Geometry check sheet. Reference: drawing and pictorial views, mm from the part's lowest x, y, z. A direction names the side the tool comes from. Coordinates: 2 decimals unless noted, no trailing zeros. Loops run counter-clockwise (first coordinate to the right, second up) from the corner with the lowest first, then second, coordinate; pieces in that order, holes last.
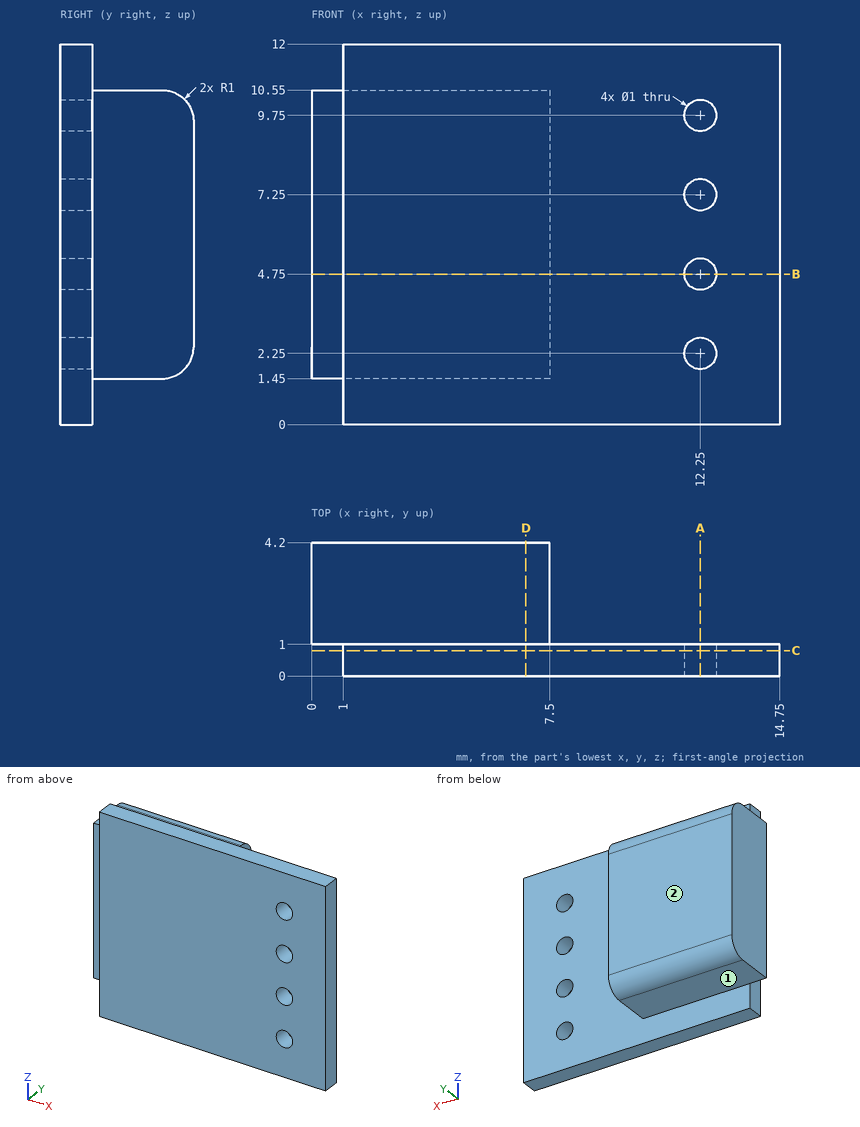
1) Access from +Z, -Z, +X, -X, +Y, -Y to the whole of each face (thin tool, end or side, straight path). Record for the marked faces 1 and 2.
Data:
face 1: -Z, +X, -X, +Y
face 2: +Z, -Z, +X, -X, +Y
2) Depth check by flat-ended pin: pin 1 (0.5 mm diameter, centred on x = 0.5, z = 6.5, fed in from -Y); pin 2 (2.5 mm diameter, centred on x = 4, y = 2.5, fed in from -Z); pin 3 (1 mm diameter, centred on x = 6.5, y = 4, fed in from -Z); pin 4 (1.1 mm diameter, centred on x = 4.5, y = 1.5, fed in from +Z). Enter the tip coordinate at first touch or a pass-through.
Data:
pin 1: stops at y = 1
pin 2: stops at z = 1.45
pin 3: stops at z = 1.5
pin 4: stops at z = 12
3) Material ranges on probe 1 along X at (y, z) = (0.5, 4.75); probe 2 along Z at (x, y) = (0.5, 1.15); probe 3 along Y at (x, z) = (13.5, 10.75), recorded low to high.
Data:
probe 1: x = 1 to 11.75, 12.75 to 14.75
probe 2: z = 1.45 to 10.55
probe 3: y = 0 to 1
4) Section check A-A on x = 12.25. Record the cut outline in (y, z).
Data:
outline: (0, 0) - (1, 0) - (1, 1.75) - (0, 1.75) - close; (0, 2.75) - (1, 2.75) - (1, 4.25) - (0, 4.25) - close; (0, 5.25) - (1, 5.25) - (1, 6.75) - (0, 6.75) - close; (0, 7.75) - (1, 7.75) - (1, 9.25) - (0, 9.25) - close; (0, 10.25) - (1, 10.25) - (1, 12) - (0, 12) - close
5) Section check C-C on y = 0.8. Record the cut outline in (x, z).
Data:
outline: (1, 0) - (14.75, 0) - (14.75, 12) - (1, 12) - close; hole circle Ø1 at (12.25, 2.25); hole circle Ø1 at (12.25, 4.75); hole circle Ø1 at (12.25, 7.25); hole circle Ø1 at (12.25, 9.75)
6) Section check D-D on x = 6.75. Record the cut outline in (y, z), and give its area (3 significant figures).
Data:
outline: (0, 0) - (1, 0) - (1, 1.45) - (3.2, 1.45) arc R1 ccw to (4.2, 2.45) - (4.2, 9.55) arc R1 ccw to (3.2, 10.55) - (1, 10.55) - (1, 12) - (0, 12) - close
area: 40.7 mm2
7) Section check B-B on z = 4.75. Record the cut outline in (x, y).
Data:
outline: (0, 1) - (1, 1) - (1, 0) - (11.75, 0) - (11.75, 1) - (7.5, 1) - (7.5, 4.2) - (0, 4.2) - close; (12.75, 0) - (14.75, 0) - (14.75, 1) - (12.75, 1) - close
